The figure shows three views and two pictorial views of one solid part (mm, origin at its lowest corner). Answer the questions. Give positions to 0.01 mm unless a question says otherwise; leave off trailing zeros. Write each loop counter-clockwise with the first axis right and the second up, starting at its lowest first coordinate (ties: lowest second). Pieces come first, ordered by that corner, then holes. Notation, with made-up numbers: (-2, 82.5) - (43, 82.5) arc R13 cw to (43, 89.5) - close; hole circle Ø8 at (22, 28.5). An arc over 180 degrees is marked (long way). Write each question's results on one line, items separated by ' | '. Start each with the question number.
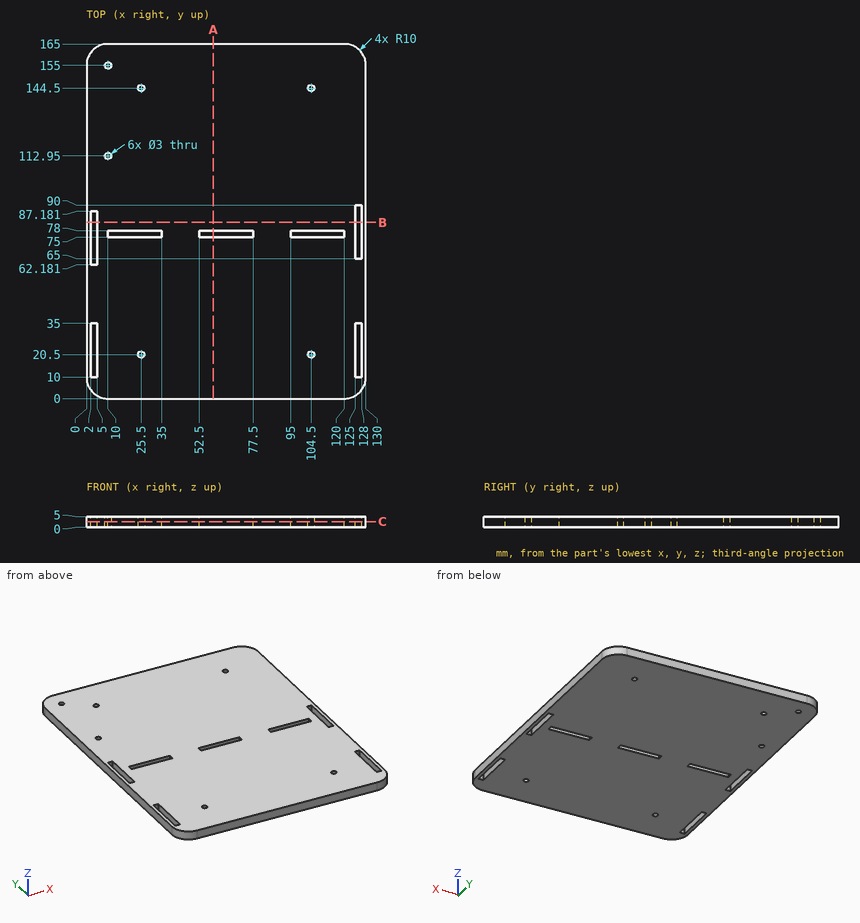
Q1. Given pin 1 (1.5 mm diameter, centred on x = 3, z = 1.5, fed in from -Y); pin 2 (1.5 mm diameter, centred on x = 126.5, z = 3, fed in from +Y), each flat-ended and moving along its own axis, determine where each tip first touches the part or whether it passes through.
Q2. A cutting plane is placed at C-C, the plane z = 2.65. Give the number of separate pieces and of enclosed holes in the cut face, and give its area (3 significant figures).
Q3. A cutting plane is placed at A-A, the plane x = 59. Write down the section's boundary in (y, z).
Q4. A cutting plane is placed at B-B, the plane y = 82. Write down the section's boundary in (x, z).
Q5. Consider L1, parallel to X at y = 144.5, z = 1; L2, parallel to Y at x = 25.5, z = 1.3; L3, parallel to X at y = 83, z = 3.5. Determine where each line is inside the solid, lowest interval first.
Result:
1) pin 1: stops at y = 2.19 | pin 2: stops at y = 163.18
2) separate pieces: 1 | enclosed holes: 13 | area: 20,800 mm2
3) outline: (0, 0) - (75, 0) - (75, 5) - (0, 5) - close; (78, 0) - (165, 0) - (165, 5) - (78, 5) - close
4) outline: (0, 0) - (2, 0) - (2, 5) - (0, 5) - close; (5, 0) - (125, 0) - (125, 5) - (5, 5) - close; (128, 0) - (130, 0) - (130, 5) - (128, 5) - close
5) L1: x = 0 to 24, 27 to 103, 106 to 130 | L2: y = 0 to 19, 22 to 75, 78 to 143, 146 to 165 | L3: x = 0 to 2, 5 to 125, 128 to 130
